Verification items for the finished model (mm, model axes). A direction names the side the tool comes from. Round coordinates to 2 decimals unless told otherwise and drop trailing zeros. Order: outer loops, then holes, each group sorted by start corner. A loop starts at its lowest first (then second) coordinate and runs counter-clockwise, first axis right, second up. Notation, with made-up numbers: M -38,57 L -6,57 A14 cw -6,73 Z; hole C 21,-17 d2. An arc over 180 degrees is marked long. One line per item, written item: value. Start each with the question number.
from build123d import *

# Parameters (mm, degrees)
SKETCH_1_W          = 94.97478029
SKETCH_1_H          = 42.97467615
SKETCH_1_W_2        = 90.97478029
SKETCH_1_H_2        = 38.97467615
EXTRUDE_1_DEPTH     = 5
SKETCH_2_W          = 9
SKETCH_2_H          = 9
EXTRUDE_2_DEPTH     = 3.4
FILLET_1_R          = 5
SKETCH_3_W          = 94.97478029
SKETCH_3_H          = 42.97467615
EXTRUDE_3_DEPTH     = 2
SKETCH_4_R          = 2.4
CUT_EXTRUDE_1_DEPTH = 3.5
SKETCH_5_R          = 1.4
CUT_EXTRUDE_2_DEPTH = 102.021837464
FILLET_2_R          = 5
FILLET_3_R          = 2
FILLET_4_R          = 2


with BuildPart() as part:
    # 草图1 → 凸台-拉伸1 (new body)
    with BuildSketch(Plane(origin=(0, 0, 1.6000508), x_dir=(-1, 0, 0), z_dir=(0, 0, -1))):
        with Locations((-45.00009017, -19.0000381)):
            Rectangle(SKETCH_1_W, SKETCH_1_H)
        with Locations((-45.00009017, -19.0000381)):
            Rectangle(SKETCH_1_W_2, SKETCH_1_H_2, mode=Mode.SUBTRACT)
    extrude(amount=EXTRUDE_1_DEPTH)

    # 草图2 → 凸台-拉伸2 (add)
    with BuildSketch(Plane(origin=(0, 0, -3.3999492), x_dir=(-1, 0, 0), z_dir=(0, 0, -1))):
        with Locations((-85.987480315, -4.012700025)):
            Rectangle(SKETCH_2_W, SKETCH_2_H)
        with Locations((-4.012700025, -4.012700025)):
            Rectangle(SKETCH_2_W, SKETCH_2_H)
        with Locations((-4.012700025, -33.987376175)):
            Rectangle(SKETCH_2_W, SKETCH_2_H)
        with Locations((-85.987480315, -33.987376175)):
            Rectangle(SKETCH_2_W, SKETCH_2_H)
    extrude(amount=-EXTRUDE_2_DEPTH)

    # 圆角1
    fillet_1_edges = [part.edges().sort_by_distance(p)[0] for p in [
        (81.487480315, -29.487376175, -1.6999492),
        (8.512700025, -29.487376175, -1.6999492),
        (8.512700025, -8.512700025, -1.6999492),
        (81.487480315, -8.512700025, -1.6999492),
    ]]
    fillet(fillet_1_edges, radius=FILLET_1_R)

    # 草图3 → 凸台-拉伸3 (add)
    with BuildSketch(Plane(origin=(0, 0, -3.3999492), x_dir=(-1, 0, 0), z_dir=(0, 0, -1))):
        with Locations((-45.00009017, -19.0000381)):
            Rectangle(SKETCH_3_W, SKETCH_3_H)
    extrude(amount=EXTRUDE_3_DEPTH)

    # 草图4 → 切除-拉伸1 (cut)
    with BuildSketch(Plane(origin=(0, 0, -5.3999492), x_dir=(-1, 0, 0), z_dir=(0, 0, -1))):
        with Locations((-86.00017272, -4.00000762)):
            Circle(SKETCH_4_R)
        with Locations((-4.00000762, -4.00000762)):
            Circle(SKETCH_4_R)
        with Locations((-4.00000762, -34.00006858)):
            Circle(SKETCH_4_R)
        with Locations((-86.00017272, -34.00006858)):
            Circle(SKETCH_4_R)
    extrude(amount=-CUT_EXTRUDE_1_DEPTH, mode=Mode.SUBTRACT)

    # 草图5 → 切除-拉伸2 (cut, through all)
    with BuildSketch(Plane(origin=(0, 0, -1.8999492), x_dir=(-1, 0, 0), z_dir=(0, 0, -1))):
        with Locations((-86.00017272, -4.00000762)):
            Circle(SKETCH_5_R)
        with Locations((-4.00000762, -4.00000762)):
            Circle(SKETCH_5_R)
        with Locations((-4.00000762, -34.00006858)):
            Circle(SKETCH_5_R)
        with Locations((-86.00017272, -34.00006858)):
            Circle(SKETCH_5_R)
    extrude(amount=-CUT_EXTRUDE_2_DEPTH, mode=Mode.SUBTRACT)

    # 圆角2
    fillet_2_edges = [part.edges().sort_by_distance(p)[0] for p in [
        (92.487480315, 2.487299975, -1.8999492),
        (-2.487299975, 2.487299975, -1.8999492),
        (-2.487299975, -40.487376175, -1.8999492),
        (92.487480315, -40.487376175, -1.8999492),
    ]]
    fillet(fillet_2_edges, radius=FILLET_2_R)

    # 圆角3
    fillet_3_edges = [part.edges().sort_by_distance(p)[0] for p in [
        (45.00009017, -40.487376175, -5.3999492),
        (92.487480315, -19.0000381, -5.3999492),
        (-2.487299975, -19.0000381, -5.3999492),
        (45.00009017, 2.487299975, -5.3999492),
        (91.023014221, 1.022833881, -5.3999492),
        (-1.022833881, 1.022833881, -5.3999492),
        (-1.022833881, -39.022910081, -5.3999492),
        (91.023014221, -39.022910081, -5.3999492),
    ]]
    fillet(fillet_3_edges, radius=FILLET_3_R)

    # 圆角4
    fillet_4_edges = [part.edges().sort_by_distance(p)[0] for p in [
        (-0.487299975, 0.487299975, 0.8000508),
        (90.487480315, 0.487299975, 0.8000508),
        (-0.487299975, -38.487376175, 0.8000508),
        (90.487480315, -38.487376175, 0.8000508),
    ]]
    fillet(fillet_4_edges, radius=FILLET_4_R)


solid = part.part
1. Section check A-A (x = 79.5). Record the cut outline in (y, z).
2. Tool access check on faces 4 (the face through (8.513, -37, -2)), 5 (the face through (2.71, -4.54, -0.96)). Record the directions out of +Z, -Z, +X, -X, +Y, -Y that give a thin tool (end or side, any length) a straight path to the whole face; none if there is none.
3. Section check C-C (z = -4.25). Record the cut outline in (x, y).
4. Section check B-B (y = -22). Record the cut outline in (x, z).
5. Depth check by flat-ended pin: pin 1 (1 mm diameter, centred on y = -36.5, z = -1.5, fed in from +X); pin 2 (1.5 mm diameter, centred on x = 34, y = -24.5, fed in from +Z); pin 3 (3 mm diameter, centred on x = 4, y = -34, fed in from -Z). Enter the tip coordinate at first touch or a pass-through.
6. Draft check along Y on faces 1 (the face through (45, 2, 1.6)), 2 (the face through (-0.984, -39.062, -0.935)), 3 (the face through (46, -38.487, -1)). Enter one of: released by +Y, released by -Y, zero draft, split by the parting line, or undercut.
7. Scan lines: line 1 along Y through (x, z) = (44.5, -1.75); line 2 along X through (y, z) = (-18, -1.5); line 3 along Y through (x, z) = (85.5, -3.5). Record each from-to range of solid material in increasing order.
Geometry check:
1. outline: M -40.49,-3.4 A2 ccw -38.49,-5.4 L 0.49,-5.4 A2 ccw 2.49,-3.4 L 2.49,1.6 L 0.49,1.6 L 0.49,-3.4 L -38.49,-3.4 L -38.49,1.6 L -40.49,1.6 Z
2. face 4: +Z
2. face 5: +Z, -Z
3. outline: M -2.3,-35.49 A4.81 ccw 2.51,-40.3 L 87.49,-40.3 A4.81 ccw 92.3,-35.49 L 92.3,-2.51 A4.81 ccw 87.49,2.3 L 2.51,2.3 A4.81 ccw -2.3,-2.51 Z; hole C 4,-34 d4.8; hole C 4,-4 d4.8; hole C 86,-34 d4.8; hole C 86,-4 d4.8
4. outline: M -2.49,-3.4 A2 ccw -0.49,-5.4 L 90.49,-5.4 A2 ccw 92.49,-3.4 L 92.49,1.6 L 90.49,1.6 L 90.49,-3.4 L -0.49,-3.4 L -0.49,1.6 L -2.49,1.6 Z
5. pin 1: stops at x = 92.46
5. pin 2: stops at z = -3.4
5. pin 3: stops at z = -1.9
6. face 1: zero draft
6. face 2: released by -Y
6. face 3: undercut
7. line 1: y = -40.49 to -38.49, 0.49 to 2.49
7. line 2: x = -2.49 to -0.49, 90.49 to 92.49
7. line 3: y = -40.48 to -36.35, -31.65 to -6.35, -1.65 to 2.48
